Read the model definition and answer for the solid it produces. Units are mm, in the model's axes. A direction names the side the tool comes from. Coordinates: 2 decimals unless noted, no trailing zeros. Write each loop counter-clockwise with the first axis right and the second up, starting at its lowest first coordinate (ties: lowest second). Pieces come first, ordered by that corner, then holes. Notation, with made-up numbers: (-27, 40.5) -> (28, 40.5) arc R15 cw to (28, 52.5) -> close; hole circle Ø10 at (-13.5, 26). An arc over 180 degrees is marked (long way). One line per item, written item: value. Start each with the question number.
from build123d import *

# Parameters (mm, degrees)
F0_R     = 1.5
F1_DEPTH = 2.3
F2_R     = 0.8


with BuildPart() as f1:
    # F0 (on Top) → F1 (new body)
    with BuildSketch(Plane.XY):
        with BuildLine():
            Line((3.872134, 14.051424), (-20.127866, 14.051424))
            ThreePointArc((-20.127866, 14.051424), (-23.6634, 12.586958), (-25.127866, 9.051424))
            Line((-25.127866, 9.051424), (-25.127866, -6.948576))
            ThreePointArc((-25.127866, -6.948576), (-23.6634, -10.48411), (-20.127866, -11.948576))
            Line((-20.127866, -11.948576), (3.872134, -11.948576))
            ThreePointArc((3.872134, -11.948576), (7.407668, -10.48411), (8.872134, -6.948576))
            Line((8.872134, -6.948576), (8.872134, 9.051424))
            ThreePointArc((8.872134, 9.051424), (7.407668, 12.586958), (3.872134, 14.051424))
        make_face()
        with Locations((-8.127866, -8.348576)):
            Circle(F0_R, mode=Mode.SUBTRACT)
        with Locations((-8.127866, 10.851424)):
            Circle(F0_R, mode=Mode.SUBTRACT)
        Polygon((3.072134, -4.748576), (-18.927866, -4.748576), (-18.927866, 7.251424), (3.072134, 7.251424), (3.072134, 3.551424), (5.072134, 3.551424), (5.072134, 1.251424), (5.072134, -1.048576), (3.072134, -1.048576), align=None, mode=Mode.SUBTRACT)
    extrude(amount=F1_DEPTH)

    # F2
    f2_edges = [f1.edges().sort_by_distance(p)[0] for p in [
        (-23.6634, -10.48411, 2.3),
    ]]
    fillet(f2_edges, radius=F2_R)


solid = f1.part
1. A cutting plane is placed at C-C on z = 0.65. Give the vertices of the cut face in (x, y), then the cut area to 3 significant figures.
2. Find the intervals of material crossed by probe 1 along Y at (x, z) = (-8, 0.5); probe 2 along Y at (x, z) = (-11.5, 0.25); probe 3 along Y at (x, z) = (-7.5, 0.9), in increasing order. Write a range as from..to.
3. A cutting plane is placed at A-A on x = -1. Give the vertices of the cut face in (y, z), then the cut area to 3 significant figures.
4. A cutting plane is placed at B-B on y = 2.5. Give the vertices of the cut face in (x, z), then the cut area to 3 significant figures.
5. For a pull along X with two mould halves and no side action, classify faces 1 (the face through (-23.62, 12.63, 0.74)), 2 (the face through (7.37, -10.52, 0.74)), 3 (the face through (-8, 14.051, 1)), 4 (the face through (-18.928, 1, 1)) as +X half, -X half, draft (parallel to the pull), parting line (faces both ways), or undercut.
6. A tool of negligible diameter and unlimited length cuts with its end or side. For faces 5 (the face through (-8.3, 13.82, 2.06)), 6 (the face through (3.072, 5, 1)), from which of +Z, -Z, +X, -X, +Y, -Y can it reach the whole face along a straight path? Write none if from no direction.
Derived:
1. outline: (-25.13, -6.95) arc R5 ccw to (-20.13, -11.95) -> (3.87, -11.95) arc R5 ccw to (8.87, -6.95) -> (8.87, 9.05) arc R5 ccw to (3.87, 14.05) -> (-20.13, 14.05) arc R5 ccw to (-25.13, 9.05) -> close; hole (-18.93, -4.75) -> (3.07, -4.75) -> (3.07, -1.05) -> (5.07, -1.05) -> (5.07, 3.55) -> (3.07, 3.55) -> (3.07, 7.25) -> (-18.93, 7.25) -> close; hole circle Ø3 at (-8.13, -8.35); hole circle Ø3 at (-8.13, 10.85)
1. area: 575 mm2
2. probe 1: y = -11.95..-9.84, -6.85..-4.75, 7.25..9.36, 12.35..14.05
2. probe 2: y = -11.95..-4.75, 7.25..14.05
2. probe 3: y = -11.95..-9.71, -6.99..-4.75, 7.25..9.49, 12.21..14.05
3. outline: (-11.95, 0) -> (-4.75, 0) -> (-4.75, 2.3) -> (-11.15, 2.3) arc R0.8 ccw to (-11.95, 1.5) -> close; (7.25, 0) -> (14.05, 0) -> (14.05, 1.5) arc R0.8 ccw to (13.25, 2.3) -> (7.25, 2.3) -> close
3. area: 31.9 mm2
4. outline: (-25.13, 0) -> (-18.93, 0) -> (-18.93, 2.3) -> (-24.33, 2.3) arc R0.8 ccw to (-25.13, 1.5) -> close; (5.07, 0) -> (8.87, 0) -> (8.87, 1.5) arc R0.8 ccw to (8.07, 2.3) -> (5.07, 2.3) -> close
4. area: 22.7 mm2
5. face 1: -X half
5. face 2: +X half
5. face 3: draft
5. face 4: undercut
6. face 5: +Z, +X, -X, +Y
6. face 6: +Z, -Z
